The drawing under review shows one solid part. Ordinate dimensions are in mm from its lowest x, y, z. Round coordinates to 2 decimals unless told otherwise and drop trailing zeros. Order: outer loops, then holes, each group sorted by start corner. A loop starts at its lowest first (then second) coordinate and runs counter-clockwise, first axis right, second up. Notation, with made-up numbers: M 24.5,19.25 L 48.5,19.25 A27 ccw 48.5,45.25 Z; hole C -34.5,35.25 d4. An arc over 180 degrees is marked long. Answer as a JSON object with one key per item and string values. Group by question number.
1. Clearance check with flat-ended pins moving along their axes: P1, Ø5, axis at x = 75, y = 7.66, coming from the +Z side; P2, Ø2, axis at y = 127.5, z = 45, coming from the -X side; P3, Ø0.9, axis at x = 7, y = 75.5, coming from the +Z side. State where each tip first meets the part, or that it passes through.
2. Add section C-C on y = 48.5. State the section outline as (x, z) points, and give its area (3 significant figures).
3. Mouldability with a two-part tool opening along X and no side actions: class the marked faces 1, 2, 3 and 4 as released by +X, released by -X, zero draft, split by the parting line, or undercut.
4. Add section A-A on z = 6. State the section outline as (x, y) points, and give its area (3 significant figures).
5. To check wall thickness, follow probe 1 along Y at (x, z) = (75, 22); probe 2 along Y at (x, z) = (74.5, 43); probe 3 along Z at (x, y) = (53, 112). State the ranges of each line that lie inside material, in increasing order. Write a range as [from, to].
6. Add section B-B on x = 49. State the section outline as (y, z) points, and give its area (3 significant figures).
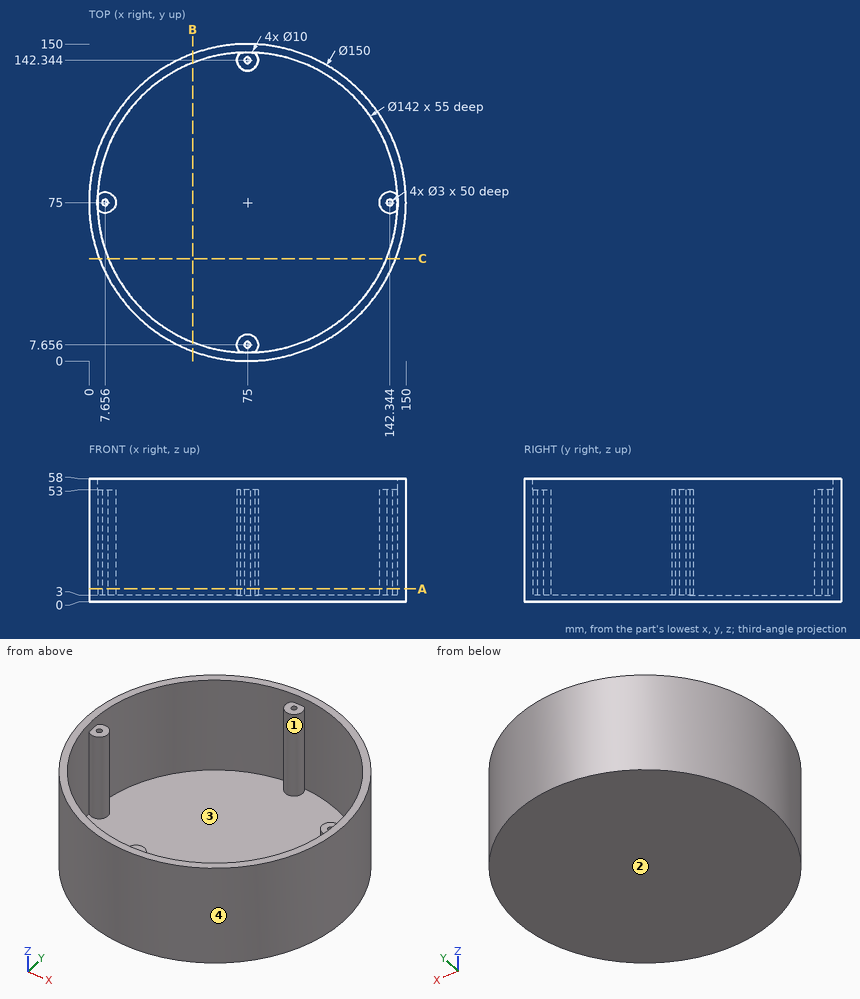
Recorded:
{
 "1": {"P1": "stops at z = 53", "P2": "stops at x = 20.48", "P3": "stops at z = 3"},
 "2": {"outline": "M 4.84,0 L 145.16,0 L 145.16,58 L 140.87,58 L 140.87,3 L 9.13,3 L 9.13,58 L 4.84,58 Z", "area": "893 mm²"},
 "3": {"face 1": "undercut", "face 2": "zero draft", "face 3": "undercut", "face 4": "split by the parting line"},
 "4": {"outline": "C 75,75 d150; hole M 4.09,71.5 A71 ccw 71.5,4.09 A5 cw long 78.5,4.09 A71 ccw 145.91,71.5 A5 cw long 145.91,78.5 A71 ccw 78.5,145.91 A5 cw long 71.5,145.91 A71 ccw 4.09,78.5 A5 cw long Z; hole C 7.66,75 d3; hole C 75,7.66 d3; hole C 75,142.34 d3; hole C 142.34,75 d3", "area": "2,090 mm²"},
 "5": {"probe 1": "y = [0, 6.16], [9.16, 12.66], [137.34, 140.84], [143.84, 150]", "probe 2": "y = [0, 6.24], [9.07, 12.63], [137.37, 140.93], [143.76, 150]", "probe 3": "z = [0, 3]"},
 "6": {"outline": "M 4.65,0 L 145.35,0 L 145.35,58 L 141.07,58 L 141.07,3 L 8.93,3 L 8.93,58 L 4.65,58 Z", "area": "893 mm²"}
}
